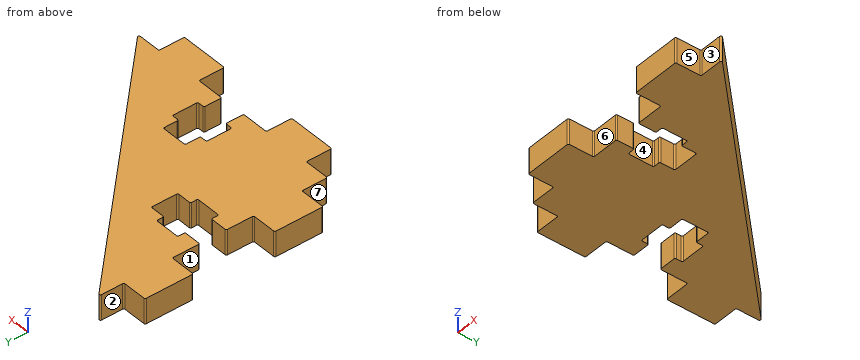
from build123d import *

# Parameters (mm, degrees)
BOSS_EXTRUDE1_DEPTH = 4.95
FILLET1_R           = 0.25
FILLET2_R           = 0.25


with BuildPart() as part:
    # Sketch2 → Boss-Extrude1 (new body)
    with BuildSketch(Plane.XY):
        Polygon((0, 45), (0, 40), (-5, 40), (-5, 30.5), (0, 30.5), (0, 25.1), (3.5, 25.1), (3.5, 26.55), (8.5, 26.55), (8.5, 25.1), (11.5, 25.1), (11.5, 19.9), (8.5, 19.9), (8.5, 18.45), (3.5, 18.45), (3.5, 19.9), (0, 19.9), (0, 14.5), (-5, 14.5), (-5, 5), (0, 5), (0, 0), (5, 0), (5, -5), (14.5, -5), (14.5, 0), (19.9, 0), (19.9, 3.5), (18.45, 3.5), (18.45, 8.5), (19.9, 8.5), (19.9, 11.5), (25.1, 11.5), (25.1, 8.5), (26.55, 8.5), (26.55, 3.5), (25.1, 3.5), (25.1, 0), (30.5, 0), (30.5, -5), (40, -5), (40, 0), (45, 0), align=None)
    extrude(amount=BOSS_EXTRUDE1_DEPTH)

    # Fillet1
    fillet1_edges = [part.edges().sort_by_distance(p)[0] for p in [
        (-5, 5, 2.475),
        (-5, 14.5, 2.475),
        (0, 19.9, 2.475),
        (0, 25.1, 2.475),
        (-5, 30.5, 2.475),
        (-5, 40, 2.475),
        (0, 45, 2.475),
        (45, 0, 2.475),
        (40, -5, 2.475),
        (30.5, -5, 2.475),
        (25.1, 0, 2.475),
        (19.9, 0, 2.475),
        (14.5, -5, 2.475),
        (5, -5, 2.475),
        (0, 0, 2.475),
    ]]
    fillet(fillet1_edges, radius=FILLET1_R)

    # Fillet2
    fillet2_edges = [part.edges().sort_by_distance(p)[0] for p in [
        (0, 5, 2.475),
        (0, 14.5, 2.475),
        (3.5, 19.9, 2.475),
        (3.5, 18.45, 2.475),
        (8.5, 18.45, 2.475),
        (8.5, 19.9, 2.475),
        (11.5, 19.9, 2.475),
        (11.5, 25.1, 2.475),
        (8.5, 25.1, 2.475),
        (8.5, 26.55, 2.475),
        (3.5, 26.55, 2.475),
        (3.5, 25.1, 2.475),
        (0, 30.5, 2.475),
        (0, 40, 2.475),
        (40, 0, 2.475),
        (30.5, 0, 2.475),
        (25.1, 3.5, 2.475),
        (26.55, 3.5, 2.475),
        (26.55, 8.5, 2.475),
        (25.1, 8.5, 2.475),
        (25.1, 11.5, 2.475),
        (19.9, 11.5, 2.475),
        (19.9, 8.5, 2.475),
        (18.45, 8.5, 2.475),
        (18.45, 3.5, 2.475),
        (19.9, 3.5, 2.475),
        (14.5, 0, 2.475),
        (5, 0, 2.475),
    ]]
    fillet(fillet2_edges, radius=FILLET2_R)


solid = part.part
Design review of the part built by this model. Coordinates are the model's own, in mm. Face numbers are marked on the shaded views. A direction names the side the tool comes from. Coordinates: 2 decimals unless noted, no trailing zeros. Order: outer loops, then holes, each group sorted by start corner. A loop starts at its lowest first (then second) coordinate and runs counter-clockwise, first axis right, second up.
Item 1: For line 1 (Y direction, x = -1.5, z = 3.9); line 2 (Y direction, x = 4, z = 1.05), list the stretches that pass through material, from the lowest coordinate up.
Item 2: Take a section at A-A, the plane x = -1. Write out the cut boundary in (y, z), then the cut area to 4 significant figures.
Item 3: For the marked faces 4, 5, 6 and 7, list the 3-axis set-ups (+Z, -Z, +X, -X, +Y, -Y) from which the entire face can be reached by the end or side of a thin tool; tool diameter is ignored.
Item 4: The part is to be moulded in two halves that separate along Y. For the marked faces 1, 2 and 3, say which applies: pulls with the +Y half, pulls with the -Y half, needs draft (parallel to the pull), parting line crosses it, or undercut.
Item 5: Take a section at B-B, the plane y = 37. Write out the cut boundary in (x, z), then the cut area to 4 significant figures.
Item 6: Take a section at C-C, the plane x = 32.5. Write out the cut boundary in (y, z).
Item 7: For pin 1 Ø0.8 at (y, z) = (25.5, 1.5) entering from -X; pin 2 Ø1.5 at (x, z) = (26.5, 1.5) entering from -Y; pin 3 Ø1.5 at (y, z) = (2.5, 1.5) entering from +X, all flat-tipped, find the tip position at first contact; note any pin that passes through.
The answers:
1. line 1: y = 5 to 14.5, 30.5 to 40
1. line 2: y = 0 to 18.45, 26.55 to 41
2. outline: (5, 0) - (14.5, 0) - (14.5, 4.95) - (5, 4.95) - close; (30.5, 0) - (40, 0) - (40, 4.95) - (30.5, 4.95) - close
2. area: 94.05 mm2
3. face 4: +Z, -Z
3. face 5: +Z, -Z, +X, -Y
3. face 6: +Z, -Z, -Y
3. face 7: +Z, -Z, -X, -Y
4. face 1: undercut
4. face 2: needs draft
4. face 3: pulls with the -Y half
5. outline: (-5, 0) - (8, 0) - (8, 4.95) - (-5, 4.95) - close
5. area: 64.35 mm2
6. outline: (-5, 0) - (12.5, 0) - (12.5, 4.95) - (-5, 4.95) - close
7. pin 1: stops at x = 0
7. pin 2: stops at y = 0
7. pin 3: stops at x = 43.25
